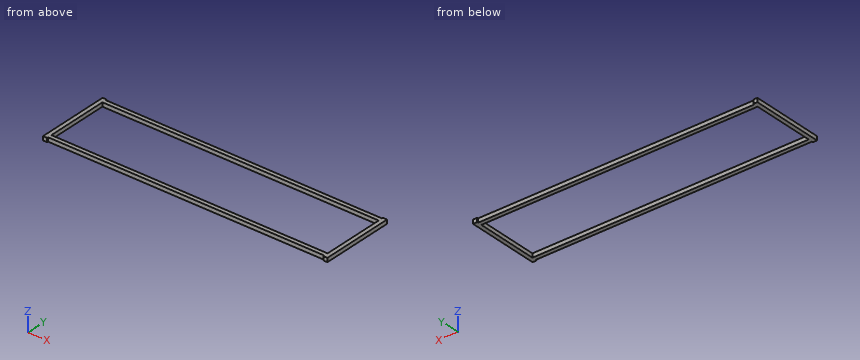
from build123d import *

# Parameters (mm, degrees)
SKETCH1_W           = 444.2968
SKETCH1_H           = 100.6475
BOSS_EXTRUDE1_DEPTH = 6.35


with BuildPart() as part:
    # Sketch1 → Boss-Extrude1 (new body)
    with BuildSketch(Plane.XY):
        Polygon((222.1484, -58.785125), (228.7016, -58.785125), (228.7016, 58.785125), (222.1484, 58.785125), (222.1484, 56.87695), (-222.1484, 56.87695), (-222.1484, 58.785125), (-228.7016, 58.785125), (-228.7016, -58.785125), (-222.1484, -58.785125), (-222.1484, -56.87695), (222.1484, -56.87695), align=None)
        Rectangle(SKETCH1_W, SKETCH1_H, mode=Mode.SUBTRACT)
    extrude(amount=BOSS_EXTRUDE1_DEPTH)


solid = part.part
Could you check a few things on this model? Use its own coordinates, in mm. Give positions to 0.01 mm unless a question says otherwise; leave off trailing zeros. Order: outer loops, then holes, each group sorted by start corner. A loop starts at its lowest first (then second) coordinate and runs counter-clockwise, first axis right, second up. Notation, with made-up numbers: (54.25, 30) - (63.25, 30) arc R24 ccw to (63.25, 48) - close; hole circle Ø9 at (36.5, 71). An arc over 180 degrees is marked (long way). One line per question, with ' | ' between items. Start each with the question number.
Item 1: I need wall thicknesses on probe 1 along X at (y, z) = (-17, 3); probe 2 along Y at (x, z) = (78.5, 1.75). Which ranges of each line are inside material? Lowest first, please. Write a range as [from, to].
Item 2: I want a section at A-A on x = -64. Write out the boundary of the cut face in (y, z), then the cut area to 3 significant figures.
Item 3: I'm going to push flat-ended pins straight in: pin 1 Ø1.9 at (x, z) = (28.5, 4) entering from -Y; pin 2 Ø1 at (x, z) = (165, 3.5) entering from +Y. Where does each tip first touch, or does it pass through?
Item 4: I want a section at C-C on z = 5.25. Write out the boundary of the cut face in (x, y).
Item 5: I want a section at B-B on y = 18.5. Write out the boundary of the cut face in (x, z), then the cut area to 3 significant figures.
Verdict:
1) probe 1: [-228.7, -222.15], [222.15, 228.7] | probe 2: [-56.88, -50.32], [50.32, 56.88]
2) outline: (-56.88, 0) - (-50.32, 0) - (-50.32, 6.35) - (-56.88, 6.35) - close; (50.32, 0) - (56.88, 0) - (56.88, 6.35) - (50.32, 6.35) - close | area: 83.2 mm^2
3) pin 1: y = -56.88 | pin 2: y = 56.88
4) outline: (-228.7, -58.79) - (-222.15, -58.79) - (-222.15, -56.88) - (222.15, -56.88) - (222.15, -58.79) - (228.7, -58.79) - (228.7, 58.79) - (222.15, 58.79) - (222.15, 56.88) - (-222.15, 56.88) - (-222.15, 58.79) - (-228.7, 58.79) - close; hole (-222.15, -50.32) - (222.15, -50.32) - (222.15, 50.32) - (-222.15, 50.32) - close
5) outline: (-228.7, 0) - (-222.15, 0) - (-222.15, 6.35) - (-228.7, 6.35) - close; (222.15, 0) - (228.7, 0) - (228.7, 6.35) - (222.15, 6.35) - close | area: 83.2 mm^2
